Geometry check sheet. Reference: drawing and pictorial views, mm from the part's lowest x, y, z. Coordinates: 2 decimals unless noted, no trailing zeros. Order: outer loops, then holes, each group sorted by start corner. A loop starts at its lowest first (then second) coordinate and runs counter-clockwise, first axis right, second up. Notation, with made-up numbers: (89, -9.5) -> (106, -9.5) arc R37 cw to (106, 29.5) -> close; hole circle Ø10 at (-22.5, 31.5). An arc over 180 degrees is marked (long way). Use CSV: the item, a comma, the result in double quotes. Start each with the question number.
1) Sectioned sample at D-D on z = 226.5. Record the boundary of the cut face in (x, y), then the cut area to 3 significant figures.
2) Sectioned sample at B-B on x = 25.4. Record the boundary of the cut face in (y, z), then the cut area to 3 significant figures.
3) Sectioned sample at C-C on x = 43. Record the boundary of the cut face in (y, z), then the cut area to 3 significant figures.
4) Sectioned sample at A-A on z = 38.1. Record the boundary of the cut face in (x, y), then the cut area to 3 significant figures.
5) Go/stop test with a flat-tipped pin: pin 1 (12.5 mm diameter, centred on x = 25.4, z = 38.1, fed in from -Y). Record where the tip stops, or that it passes through.
6) Release check for a two-part mould opening along Z. For the marked faces 1, 2, 3 and 4 record: released by +Z, released by -Z, zero draft, split by the parting line, or undercut.
7) Scan lines: line 1 along Z through (x, y) = (25.4, 22.25); line 2 along Z through (x, y) = (25, 22); line 3 along X through (y, z) = (21, 38). Record each from-to range of solid material in increasing order.
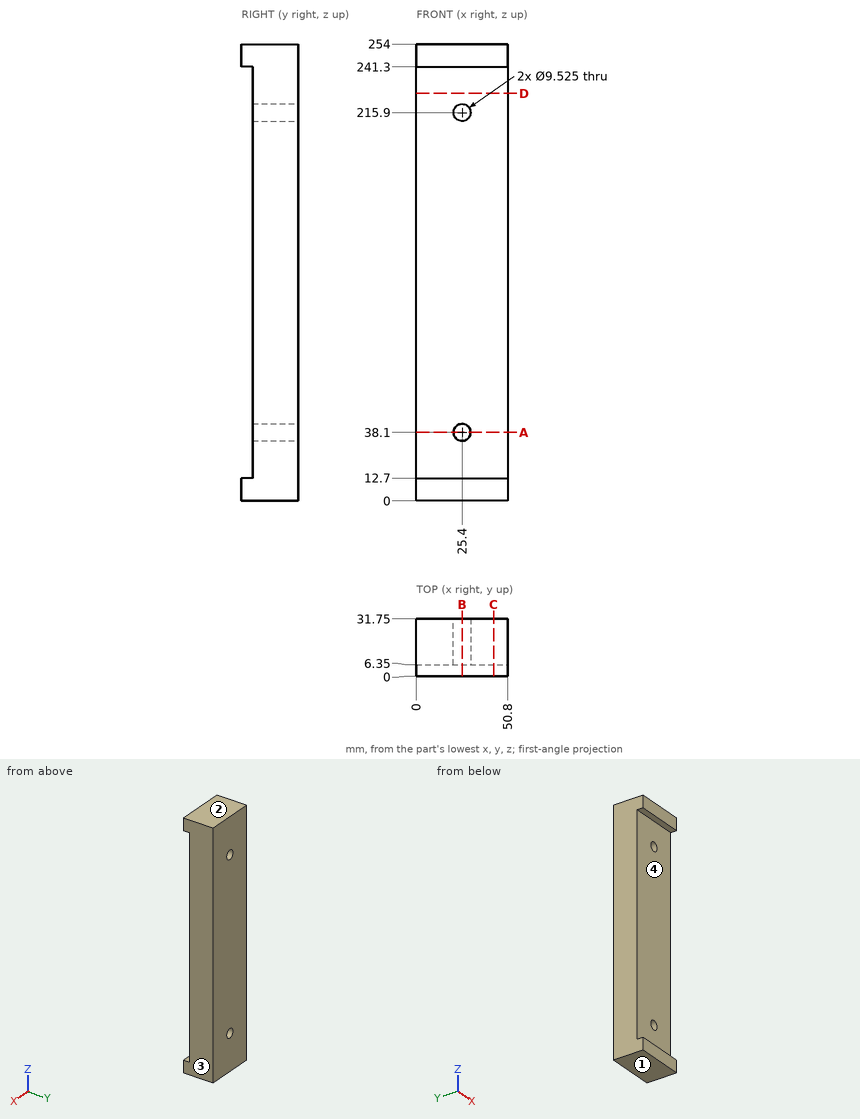
Answers follow:
1,outline,"(0, 6.35) -> (50.8, 6.35) -> (50.8, 31.75) -> (0, 31.75) -> close"
1,area,"1,290 mm²"
2,outline,"(0, 0) -> (31.75, 0) -> (31.75, 33.34) -> (6.35, 33.34) -> (6.35, 12.7) -> (0, 12.7) -> close; (0, 241.3) -> (6.35, 241.3) -> (6.35, 220.66) -> (31.75, 220.66) -> (31.75, 254) -> (0, 254) -> close; (6.35, 42.86) -> (31.75, 42.86) -> (31.75, 211.14) -> (6.35, 211.14) -> close"
2,area,"6,130 mm²"
3,outline,"(0, 0) -> (31.75, 0) -> (31.75, 254) -> (0, 254) -> (0, 241.3) -> (6.35, 241.3) -> (6.35, 12.7) -> (0, 12.7) -> close"
3,area,"6,610 mm²"
4,outline,"(0, 6.35) -> (20.64, 6.35) -> (20.64, 31.75) -> (0, 31.75) -> close; (30.16, 6.35) -> (50.8, 6.35) -> (50.8, 31.75) -> (30.16, 31.75) -> close"
4,area,"1,050 mm²"
5,pin 1,"stops at y = 6.35"
6,face 1,"released by -Z"
6,face 2,"released by +Z"
6,face 3,"zero draft"
6,face 4,"undercut"
7,line 1,"z = 0 to 33.34, 42.86 to 211.14, 220.66 to 254"
7,line 2,"z = 0 to 33.35, 42.85 to 211.15, 220.65 to 254"
7,line 3,"x = 0 to 20.64, 30.16 to 50.8"
